Here's the drawing with two shaded views (mm, measured from the low corner). I have some questions. Coordinates: 2 decimals unless noted, no trailing zeros. Write each loop counter-clockwise with the first axis right and the second up, starting at its lowest first coordinate (ties: lowest second). Pieces come first, ordered by that corner, then holes. Notation, with made-up numbers: (18, 76) -> (42, 76) arc R16 cw to (42, 96) -> close; hole circle Ø11 at (73.25, 85). An arc over 180 degrees is marked (long way). Put each result on its own line as item: value. Start each with the question number.
Item 1: I want a section at A-A, the plane z = 74.5. List the corners of the cut face in (x, y) for me, then the cut area to 3 significant figures.
Item 2: I want a section at C-C, the plane y = 6.25. List the corners of the cut face in (x, z) for me, then the cut area to 3 significant figures.
Item 3: I want a section at B-B, the plane x = 74.5. List the corners of the cut face in (y, z) for me, then the cut area to 3 significant figures.
Item 4: If we mould it in two halves opening along Z, with no side actions, what happens to the marked faces 1 and 2? For each: released by +Z, released by -Z, zero draft, split by the parting line, or undercut.
Item 5: I need wall thicknesses on line 1 (Z direction, x = 74.5, y = 8.2); line 2 (Z direction, x = 74.5, y = 3.25); line 3 (X direction, y = 9.75, z = 75.5). Which ranges of each line are inside material? Lowest first, please. Write a range as [from, to].
Item 6: For pin 1 (4 mm diameter, centred on x = 21, y = 9, fed in from +Z); pin 2 (4 mm diameter, centred on y = 6, z = 71, fed in from -X); pin 3 (1.5 mm diameter, centred on x = 42, z = 33, fed in from +Y), each with a flat end and sliding along its axis, tell me the tip position at first contact or that it passes through.
Item 7: I want a section at D-D, the plane x = 122.5. List the corners of the cut face in (y, z) for me, then the cut area to 3 significant figures.
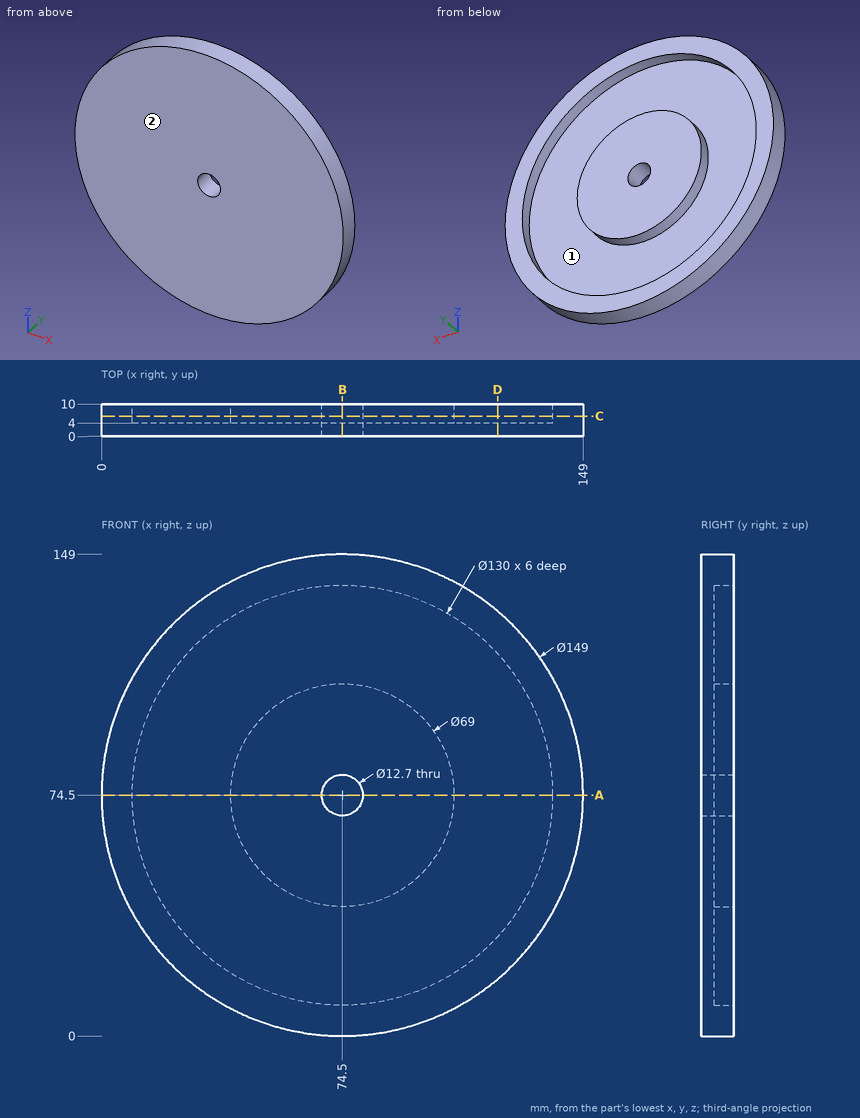
Calculated:
1. outline: (0, 0) -> (68.15, 0) -> (68.15, 10) -> (40, 10) -> (40, 4) -> (9.5, 4) -> (9.5, 10) -> (0, 10) -> close; (80.85, 0) -> (149, 0) -> (149, 10) -> (139.5, 10) -> (139.5, 4) -> (109, 4) -> (109, 10) -> (80.85, 10) -> close
1. area: 997 mm2
2. outline: circle Ø149 at (74.5, 74.5); circle Ø69 at (74.5, 74.5); hole circle Ø130 at (74.5, 74.5); hole circle Ø12.7 at (74.5, 74.5)
2. area: 7,780 mm2
3. outline: (0, 0) -> (10, 0) -> (10, 9.5) -> (4, 9.5) -> (4, 40) -> (10, 40) -> (10, 68.15) -> (0, 68.15) -> close; (0, 80.85) -> (10, 80.85) -> (10, 109) -> (4, 109) -> (4, 139.5) -> (10, 139.5) -> (10, 149) -> (0, 149) -> close
3. area: 997 mm2
4. face 1: undercut
4. face 2: zero draft
5. line 1: z = [0, 9.5], [40, 68.15], [80.85, 109], [139.5, 149]
5. line 2: z = [0, 68.15], [80.85, 149]
5. line 3: x = [0.01, 9.51], [40.01, 68.23], [80.77, 108.99], [139.49, 148.99]
6. pin 1: stops at z = 128.33
6. pin 2: stops at x = 0.02
6. pin 3: stops at y = 4
7. outline: (0, 17.52) -> (10, 17.52) -> (10, 30.67) -> (4, 30.67) -> (4, 118.33) -> (10, 118.33) -> (10, 131.48) -> (0, 131.48) -> close
7. area: 614 mm2
